The model under review builds one solid part; all positions refer to its coordinate system, in mm. Coordinates: 2 decimals unless noted, no trailing zeros. Loops run counter-clockwise (first coordinate to the right, second up) from the corner with the lowest first, then second, coordinate; pieces in that order, holes last. Notation, with made-up numbers: M -22,25.25 L 21,25.25 A18 cw 21,36.25 Z; hole C 19.5,89 d8. An arc over 180 degrees is marked long. Return JSON: item names as keys, results as strings.
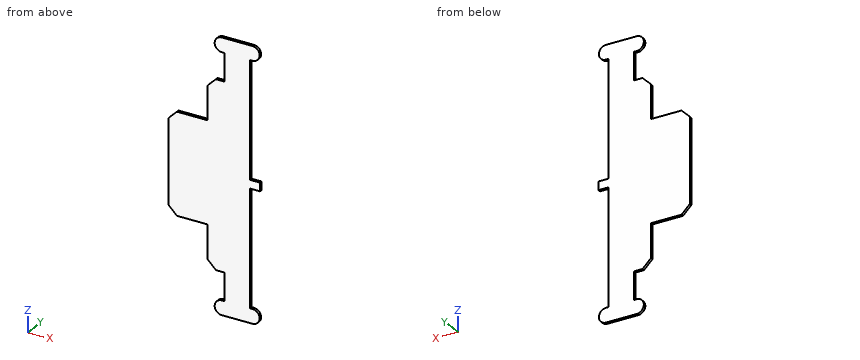
Autodesk Inventor part; units mm, degrees
ref_plane "YZ Plane" through (0, 0, 0) normal (1, 0, 0) x (0, 1, 0)
ref_plane "XZ Plane" through (0, 0, 0) normal (0, 1, 0) x (-1, 0, 0)
ref_plane "XY Plane" through (0, 0, 0) normal (0, 0, 1) x (1, 0, 0)
sketch "Sketch1" plane through (0, 0, 0) normal (0, 1, 0) x (-1, 0, 0)
  line L0 (7.5, 80) -> (-7.5, 80)
  line L1 (-7.5, -80) -> (7.5, -80)
  line L2 (7.5, 75.75) -> (7.85, 75.75)
  line L3 (7.5, 80) -> (9, 80)
  line L4 (7.5, 71.5) -> (9, 71.5)
  arc A0 (9, 71.5) -> (9, 80) centre (9, 75.75) ccw
  line L5 (7.5, 74.6) -> (9, 74.6)
  line L6 (7.5, 76.9) -> (9, 76.9)
  arc A1 (9, 74.6) -> (9, 76.9) centre (9, 75.75) ccw
  line L7 (7.5, 0) -> (-7.5, 0) construction
  line L8 (-7.5, 80) -> (-9, 80)
  line L9 (-7.5, 71.5) -> (-9, 71.5)
  arc A2 (-9, 80) -> (-9, 71.5) centre (-9, 75.75) ccw
  line L10 (-7.5, 74.6) -> (-9, 74.6)
  line L11 (-7.5, 76.9) -> (-9, 76.9)
  arc A3 (-9, 76.9) -> (-9, 74.6) centre (-9, 75.75) ccw
  line L12 (7.5, -80) -> (9, -80)
  line L13 (7.5, -71.5) -> (9, -71.5)
  arc A4 (9, -80) -> (9, -71.5) centre (9, -75.75) ccw
  line L14 (7.5, -74.6) -> (9, -74.6)
  line L15 (7.5, -76.9) -> (9, -76.9)
  arc A5 (9, -76.9) -> (9, -74.6) centre (9, -75.75) ccw
  arc A6 (-9, -71.5) -> (-9, -80) centre (-9, -75.75) ccw
  line L16 (-7.5, -71.5) -> (-9, -71.5)
  line L17 (-7.5, -74.6) -> (-9, -74.6)
  arc A7 (-9, -74.6) -> (-9, -76.9) centre (-9, -75.75) ccw
  line L18 (-7.5, -76.9) -> (-9, -76.9)
  line L19 (-7.5, -80) -> (-9, -80)
  line L20 (7.5, 55) -> (12.5, 55)
  line L21 (17.5, 50) -> (17.5, 30)
  line L22 (17.5, 30) -> (35.5, 30)
  line L23 (40.5, 25) -> (40.5, 0)
  line L24 (7.5, -55) -> (12.5, -55)
  line L25 (17.5, -50) -> (17.5, -30)
  line L26 (17.5, -30) -> (35.5, -30)
  line L27 (40.5, -25) -> (40.5, 0)
  line L28 (12.5, 55) -> (17.5, 50)
  line L29 (35.5, 30) -> (40.5, 25)
  line L30 (40.5, -25) -> (35.5, -30)
  line L31 (17.5, -50) -> (12.5, -55)
  circle A8 centre (33.5, 0) radius 1.025
  circle A9 centre (-11.5, 0) radius 1.025
  line L32 (-7.5, 2.5) -> (-13.5, 2.5)
  line L33 (-13.5, 2.5) -> (-13.5, -2.5)
  line L34 (-13.5, -2.5) -> (-7.5, -2.5)
  line L35 (7.5, -76.9) -> (7.5, -74.6)
  line L36 (7.5, -71.5) -> (7.5, -55)
  line L37 (-7.5, -2.5) -> (-7.5, -71.5)
  line L38 (-7.5, -74.6) -> (-7.5, -76.9)
  line L39 (7.5, 55) -> (7.5, 71.5)
  line L40 (7.5, 74.6) -> (7.5, 76.9)
  line L41 (-7.5, 76.9) -> (-7.5, 74.6)
  line L42 (-7.5, 71.5) -> (-7.5, 2.5)
  point P0 (0, 0)
  point P1 (0, 0)
  point P2 (8.25, 71.5)
  point P3 (17.5, 55)
  point P4 (40.5, 30)
  point P5 (17.5, -55)
  point P6 (40.5, -30)
  dimension "d0" = 160
  dimension "d2" = 1.5
  dimension "d3" = 4.25
  dimension "d5" = 4.25
  dimension "d6" = 4.25
  dimension "d7" = 1.15
  dimension "d8" = 1.15
  dimension "d9" = 1.15
  dimension "d10" = 10
  dimension "d11" = 25
  dimension "d12" = 23
  dimension "d13" = 25
  dimension "d14" = 25
  dimension "d15" = 5
  dimension "d16" = 5
  dimension "d17" = 5
  dimension "d18" = 5
  dimension "d19" = 5
  dimension "d20" = 5
  dimension "d21" = 5
  dimension "d22" = 5
  dimension "d24" = 2.05
  dimension "d25" = 7
  dimension "d26" = 2.05
extrude "Extrusion1" add sketch "Sketch1" along normal blind 1.5 contours L3 A0 L4 L39 L20 L28 L21 L22 L29 L23 L27 L30 L26 L25 L31 L24 L36 L13 A4 L12 L1 L19 A6 L16 L37 L34 L33 L32 L42 L9 A2 L8 L0 | L40 L6 A1 L5 | L10 A3 L11 L41 | L14 A5 L15 L35 | L38 L18 A7 L17 | A8 | A9
properties part number "linefollower_chassy_model_3"
1. To check wall thickness, follow line 1 (Z direction, x = 9, y = 0.6); line 2 (X direction, y = 0.7, z = -60.5); line 3 (Z direction, x = -31.5, y = 0.7). State the ranges of each line that lie inside material, in increasing order.
Check values:
{"line 1": "-80 to -71.5, -2.5 to 2.5, 71.5 to 80", "line 2": "-7.5 to 7.5", "line 3": "-30 to 30"}
2. Add section C-C on x = -24. Give the boundary of the cut face in (y, z), plus the area to 3 significant figures.
Check values:
{"outline": "M 0,-30 L 1.5,-30 L 1.5,30 L 0,30 Z", "area": "90.0 mm²"}
3. Insertion check: pin 1 Ø0.8 at (y, z) = (0.5, 36) entering from -X; pin 2 Ø0.8 at (y, z) = (0.5, -23.5) entering from +X; pin 3 Ø0.8 at (x, y) = (10, 1) entering from -Z. Each pin has a flat end and moves straight along its axis. Give the tip position at first contact, or say it passes through.
Check values:
{"pin 1": "x = -17.5", "pin 2": "x = 7.5", "pin 3": "z = -79.96"}
4. Add section B-B on z = 9.5. Give the boundary of the cut face in (x, y), plus the area to 3 significant figures.
Check values:
{"outline": "M -40.5,0 L 7.5,0 L 7.5,1.5 L -40.5,1.5 Z", "area": "72.0 mm²"}
5. Add section A-A on y = 1.15. Give the boundary of the cut face in (x, z), plus the area to 3 significant figures.
Check values:
{"outline": "M -40.5,-25 L -35.5,-30 L -17.5,-30 L -17.5,-50 L -12.5,-55 L -7.5,-55 L -7.5,-71.5 L -9,-71.5 A4.25 ccw -9,-80 L 9,-80 A4.25 ccw 9,-71.5 L 7.5,-71.5 L 7.5,-2.5 L 13.5,-2.5 L 13.5,2.5 L 7.5,2.5 L 7.5,71.5 L 9,71.5 A4.25 ccw 9,80 L -9,80 A4.25 ccw -9,71.5 L -7.5,71.5 L -7.5,55 L -12.5,55 L -17.5,50 L -17.5,30 L -35.5,30 L -40.5,25 Z", "area": "5,020 mm²"}
